from build123d import *

# Parameters (mm, degrees)
F0_R     = 4.5
F0_R_2   = 8.5
F1_DEPTH = 10
F2_R     = 5


with BuildPart() as f1:
    # F0 (on Top) → F1 (new body)
    with BuildSketch(Plane.XY):
        with BuildLine():
            Line((-62.5, 10), (-90, 10))
            Line((-90, 10), (-90, -10))
            Line((-90, -10), (-62.5, -10))
            Line((-62.5, -10), (-17.320508, -10))
            ThreePointArc((-17.320508, -10), (-20, 0), (-17.320508, 10))
            Line((-17.320508, 10), (-62.5, 10))
        make_face()
        with Locations((-75, 0)):
            Circle(F0_R, mode=Mode.SUBTRACT)
        with BuildLine():
            Line((-3.242331, 19.735432), (-62.5, 10))
            Line((-62.5, 10), (-17.320508, 10))
            ThreePointArc((-17.320508, 10), (-11.375511, 16.449856), (-3.242331, 19.735432))
        make_face()
        with BuildLine():
            ThreePointArc((-3.242331, 19.735432), (-11.375511, 16.449856), (-17.320508, 10))
            Line((-17.320508, 10), (17.320508, 10))
            ThreePointArc((17.320508, 10), (11.375511, 16.449856), (3.242331, 19.735432))
            ThreePointArc((3.242331, 19.735432), (0, 20), (-3.242331, 19.735432))
        make_face()
        with BuildLine():
            Line((-17.320508, -10), (-62.5, -10))
            Line((-62.5, -10), (-3.242331, -19.735432))
            ThreePointArc((-3.242331, -19.735432), (-11.375511, -16.449856), (-17.320508, -10))
        make_face()
        with BuildLine():
            ThreePointArc((3.242331, 19.735432), (11.375511, 16.449856), (17.320508, 10))
            Line((17.320508, 10), (62.5, 10))
            Line((62.5, 10), (3.242331, 19.735432))
        make_face()
        with BuildLine():
            Line((62.5, 10), (17.320508, 10))
            ThreePointArc((17.320508, 10), (19.318517, 5.176381), (20, 0))
            ThreePointArc((20, 0), (19.318517, -5.176381), (17.320508, -10))
            Line((17.320508, -10), (62.5, -10))
            Line((62.5, -10), (90, -10))
            Line((90, -10), (90, 10))
            Line((90, 10), (62.5, 10))
        make_face()
        with Locations((75, 0)):
            Circle(F0_R, mode=Mode.SUBTRACT)
        with BuildLine():
            Line((17.320508, -10), (-17.320508, -10))
            ThreePointArc((-17.320508, -10), (-11.375511, -16.449856), (-3.242331, -19.735432))
            ThreePointArc((-3.242331, -19.735432), (0, -20), (3.242331, -19.735432))
            ThreePointArc((3.242331, -19.735432), (11.375511, -16.449856), (17.320508, -10))
        make_face()
        with BuildLine():
            Line((62.5, -10), (17.320508, -10))
            ThreePointArc((17.320508, -10), (11.375511, -16.449856), (3.242331, -19.735432))
            Line((3.242331, -19.735432), (62.5, -10))
        make_face()
        with BuildLine():
            Line((17.320508, 10), (-17.320508, 10))
            ThreePointArc((-17.320508, 10), (-20, 0), (-17.320508, -10))
            Line((-17.320508, -10), (17.320508, -10))
            ThreePointArc((17.320508, -10), (19.318517, -5.176381), (20, 0))
            ThreePointArc((20, 0), (19.318517, 5.176381), (17.320508, 10))
        make_face()
        Circle(F0_R_2, mode=Mode.SUBTRACT)
    extrude(amount=F1_DEPTH)

    # F2
    f2_edges = [f1.edges().sort_by_distance(p)[0] for p in [
        (-90, -10, 5),
        (-90, 10, 5),
        (90, -10, 5),
        (90, 10, 5),
    ]]
    fillet(f2_edges, radius=F2_R)


solid = f1.part
Input: part model. Units: mm. Frame: model coordinates. A direction names the side the tool comes from. Coordinates: 2 decimals unless noted, no trailing zeros. Order: outer loops, then holes, each group sorted by start corner. A loop starts at its lowest first (then second) coordinate and runs counter-clockwise, first axis right, second up. Notation, with made-up numbers: M -11,8 L 10,8 A9 ccw 10,23 Z; hole C 85,30 d7. An arc over 180 degrees is marked long. Write item = value, one per line. Start each with the question number.
(1) Section A-A on y = 0. Output: boundary loops of the cut face in (x, z).
(2) Section D-D on x = 0. Output: boundary loops of the cut face in (y, z).
(3) Pull-direction query (X, two-part tool) for faces 1 (the cylindrical face through (-89, 8, 5)), 2 (the cylindrical face through (79.16, -1.72, 4.93)), 3 (the flat face through (-1, -9, 10)); classes: released by +X, released by -X, zero draft, split by the parting line, or undercut.
(4) Section B-B on x = -75. Output: boundary loops of the cut face in (y, z), and give its area (3 significant figures).
(5) First-contact query: P1, Ø5, axis at x = -57, z = 6, coming from the +Y side; P2, Ø6, axis at x = 22, z = 3.5, coming from the +Y side; P3, Ø3, axis at x = -72, z = 6, coming from the +Y side. Flat tips, straight axial feed; report the tip coordinate or a pass-through.
(6) Line query: line 1 along Y through (x, z) = (75, 6); line 2 along X through (y, z) = (0.5, 1.5); line 3 along X through (y, z) = (-4, 7). Output: solid intervals per line, ascending. Write a range as [from, to].
(7) Reachability of faces 4 (the flat face through (74, 10, 5)), 5 (the flat face through (74, -10, 5)), 6 (the flat face through (-74, 10, 5)) from +Z, -Z, +X, -X, +Y, -Y: full face, straight path, thin tool, end or side. Return the list, or none.
(8) Section C-C on z = 2.75. Output: boundary loops of the cut face in (x, y), and give its area (3 significant figures).
Result set:
q1.outline = M -90,0 L -79.5,0 L -79.5,10 L -90,10 Z; M -70.5,0 L -8.5,0 L -8.5,10 L -70.5,10 Z; M 8.5,0 L 70.5,0 L 70.5,10 L 8.5,10 Z; M 79.5,0 L 90,0 L 90,10 L 79.5,10 Z
q2.outline = M -20,0 L -8.5,0 L -8.5,10 L -20,10 Z; M 8.5,0 L 20,0 L 20,10 L 8.5,10 Z
q3.face_1 = released by -X
q3.face_2 = undercut
q3.face_3 = zero draft
q4.outline = M -10,0 L -4.5,0 L -4.5,10 L -10,10 Z; M 4.5,0 L 10,0 L 10,10 L 4.5,10 Z
q4.area = 110 mm²
q5.P1 = 11.31
q5.P2 = 17.15
q5.P3 = 10
q6.line_1 = [-10, -4.5], [4.5, 10]
q6.line_2 = [-90, -79.47], [-70.53, -8.49], [8.49, 70.53], [79.47, 90]
q6.line_3 = [-90, -77.06], [-72.94, -7.5], [7.5, 72.94], [77.06, 90]
q7.face_4 = +Z, -Z, +X, +Y
q7.face_5 = +Z, -Z, +X, -Y
q7.face_6 = +Z, -Z, -X, +Y
q8.outline = M -90,-5 A5 ccw -85,-10 L -62.5,-10 L -3.24,-19.74 A20 ccw 3.24,-19.74 L 62.5,-10 L 85,-10 A5 ccw 90,-5 L 90,5 A5 ccw 85,10 L 62.5,10 L 3.24,19.74 A20 ccw -3.24,19.74 L -62.5,10 L -85,10 A5 ccw -90,5 Z; hole C -75,0 d9; hole C 0,0 d17; hole C 75,0 d9
q8.area = 4,510 mm²
